The model under review builds one solid part; all positions refer to its coordinate system, in mm. Face numbers are marked on the shaded views. A direction names the side the tool comes from. Round coordinates to 2 decimals unless told otherwise and drop trailing zeros. Write each loop counter-clockwise with the first axis right and the second up, starting at its lowest first coordinate (ties: lowest second). Pieces come first, ordered by that corner, then holes. Notation, with made-up numbers: (71.5, -8) -> (111.5, -8) arc R12 cw to (111.5, 8) -> close; hole circle Ø1 at (73.25, 16). An arc over 180 degrees is marked (long way). Return JSON: item names as keys, results as strings. Group by question number.
1. Mouldability with a two-part tool opening along X and no side actions: class the marked faces 4, 5 and 6 as pulls with the +X half, pulls with the -X half, needs draft (parallel to the pull), parting line crosses it, or undercut.
2. Clearance check with flat-ended pins moving along their axes: P1, Ø8, axis at x = -21.5, y = 5, coming from the -Z side; P2, Ø5.5, axis at x = 24, z = 38, coming from the +Y side; P3, Ø8, axis at x = 21, y = 24.5, coming from the -Z side; P4, Ø0.9, axis at x = -5.5, z = 2, coming from the +Y side. State where each tip first meets the part, or that it passes through.
3. Take a section at D-D, the plane z = 20.5. Write out the cut boundary in (x, y).
4. Take a section at B-B, the plane y = 0. Write out the cut boundary in (x, z).
5. Take a section at A-A, the plane x = 23.25. Write out the cut boundary in (y, z).
6. For line 1 along X through (y, z) = (6.5, 9); line 2 along Y through (x, z) = (23.25, 38.3); line 3 along Y through (x, z) = (-22.25, 36.1), list the stretches that pass through material, from the lowest coordinate up. Write a range as from..to.
7. Tool access review of the marked faces 1, 2 and 3: name each direction out of +Z, -Z, +X, -X, +Y, -Y from which nothing blocks a thin tool from reaching the whole face with its end or side.
8. Take a section at C-C, the plane z = 7.5. Write out the cut boundary in (x, y).
Autodesk Inventor part; units mm, degrees
ref_plane "YZ Plane" through (0, 0, 0) normal (1, 0, 0) x (0, 1, 0)
ref_plane "XZ Plane" through (0, 0, 0) normal (0, 1, 0) x (-1, 0, 0)
ref_plane "XY Plane" through (0, 0, 0) normal (0, 0, 1) x (1, 0, 0)
sketch "Sketch1" plane through (0, 0, 0) normal (0, 0, 1) x (1, 0, 0)
  point P0 (0, 0)
sketch "Sketch2" plane through (0, 0, 0) normal (0, 0, 1) x (1, 0, 0)
  line L0 (-14.25, -53.5) -> (14.25, -53.5)
  line L1 (14.25, -53.5) -> (14.25, 53.5)
  line L2 (14.25, 53.5) -> (-14.25, 53.5)
  line L3 (-14.25, 53.5) -> (-14.25, -53.5)
  line L4 (-14.25, -53.5) -> (14.25, 53.5) construction
  line L5 (14.25, -53.5) -> (-14.25, 53.5) construction
  line L6 (14.25, -53.5) -> (17.25, -53.5)
  line L7 (17.25, -53.5) -> (17.25, 53.5)
  line L8 (17.25, 53.5) -> (14.25, 53.5)
  line L9 (14.25, 53.5) -> (14.25, -53.5)
  line L10 (-14.25, -53.5) -> (-17.25, -53.5)
  line L11 (-17.25, -53.5) -> (-17.25, 53.5)
  line L12 (-17.25, 53.5) -> (-14.25, 53.5)
  line L13 (-14.25, 53.5) -> (-14.25, -53.5)
  line L14 (-17.25, 53.5) -> (17.25, 53.5)
  line L15 (17.25, 53.5) -> (17.25, 56.5)
  line L16 (17.25, 56.5) -> (-17.25, 56.5)
  line L17 (-17.25, 56.5) -> (-17.25, 53.5)
  point P0 (0, 0)
  dimension "d0" = 28.5
  dimension "d1" = 107
  dimension "d2" = 3
  dimension "d3" = 3
  dimension "d4" = 107
  dimension "d5" = 3
extrude "Extrusion1" add sketch "Sketch2" along normal blind 40 contours L10 L11 L12 L3 | L1 L8 L7 L6 | L12 L17 L16 L15 L8 L2
extrude "Extrusion2" add sketch "Sketch2" along normal blind 3 contours L3 L2 L1 L0
ref_plane "Work Plane1" through (-17.25, -53.5, 0) normal (-1, 0, 0) x (0, 0, 1)
sketch "Sketch3" plane through (-17.25, -53.5, 0) normal (-1, 0, 0) x (0, 0, 1)
  line L0 (0, 110) -> (40, 110)
  line L1 (0, 0) -> (40, 0)
  line L2 (40, 110) -> (35, 110)
  line L3 (35, 110) -> (35, 0)
  line L4 (35, 0) -> (40, 0)
  line L5 (40, 0) -> (40, 110)
  point P0 (0, 53.5)
  dimension "d11" = 5
extrude "Extrusion3" add sketch "Sketch3" along normal blind 10
ref_plane "Work Plane2" through (17.25, -53.5, 0) normal (1, 0, 0) x (0, 0, -1)
sketch "Sketch4" plane through (17.25, -53.5, 0) normal (1, 0, 0) x (0, 0, -1)
  line L0 (-40, 0) -> (-40, 110)
  line L1 (-40, 0) -> (-35, 0)
  line L2 (-35, 0) -> (-35, 108.8698)
  line L3 (-35, 108.8698) -> (-40, 108.8698)
  line L4 (-40, 108.8698) -> (-40, 0)
  point P0 (0, 53.5)
  dimension "d15" = 5
extrude "Extrusion4" add sketch "Sketch4" along normal blind 10
ref_plane "Work Plane3" through (-14.25, 53.5, 40) normal (0, -1, 0) x (1, 0, 0)
sketch "Sketch5" plane through (-14.25, 53.5, 40) normal (0, -1, 0) x (1, 0, 0)
  line L0 (0, -37) -> (28.5, -37)
  line L1 (28.5, -37) -> (28.5, 0)
  line L2 (0, -37) -> (28.5, -37)
  line L3 (28.5, -37) -> (28.5, -22)
  line L4 (28.5, -22) -> (0, -22)
  line L5 (0, -22) -> (0, -37)
  line L6 (31.5, 0) -> (-13, 0)
  line L7 (0, 0) -> (28.5, 0)
  line L8 (28.5, 0) -> (28.5, -10)
  line L9 (28.5, -10) -> (0, -10)
  line L10 (0, -10) -> (0, 0)
  point P0 (14.25, -40)
  dimension "d19" = 15
  dimension "d20" = 10
extrude "Extrusion5" cut sketch "Sketch5" against normal blind 10 contours L5 L4 L1 L0
extrude "Extrusion6" cut sketch "Sketch5" against normal blind 10 contours L9 L10 L6 L1
ref_plane "Work Plane4" through (0, 0, 0) normal (0, 0, -1) x (-1, 0, 0)
sketch "Sketch6" plane through (0, 0, 0) normal (0, 0, -1) x (-1, 0, 0)
  line L0 (-14.25, 53.5) -> (-14.25, 56.5)
  line L1 (14.25, -53.5) -> (14.25, 56.5)
  line L2 (-14.25, 56.5) -> (14.25, 56.5)
  line L3 (14.25, 56.5) -> (14.25, 46.5)
  line L4 (14.25, 46.5) -> (-14.25, 46.5)
  line L5 (-14.25, 46.5) -> (-14.25, 56.5)
  point P0 (0, 0)
  point P1 (14.25, 56.5)
  dimension "d26" = 10
extrude "Extrusion7" cut sketch "Sketch6" against normal blind 10
ref_plane "Work Plane5" through (0, 0, 40) normal (0, 0, 1) x (1, 0, 0)
ref_plane "Work Plane6" through (0, 0, 40) normal (0, 0, 1) x (1, 0, 0)
sketch "Sketch7" plane through (0, 0, 40) normal (0, 0, 1) x (1, 0, 0)
  circle A0 centre (23.25, 0) radius 1.75
  point P0 (0, 0)
  dimension "d31" = 3.5
sketch "Sketch8" plane through (0, 0, 40) normal (0, 0, 1) x (1, 0, 0)
  circle A0 centre (-22.25, 0) radius 1.75
  point P0 (0, 0)
  dimension "d32" = 3.5
extrude "Extrusion8" cut sketch "Sketch8" against normal blind 10
extrude "Extrusion9" cut sketch "Sketch7" against normal blind 10
properties part number "suport_batterie_2"
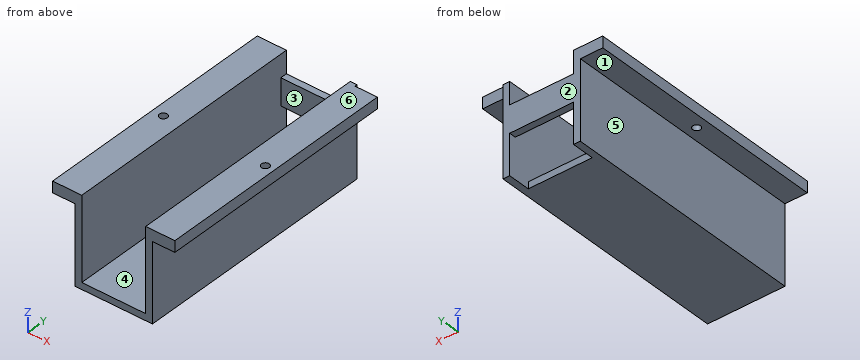
Output:
{
 "1": {"face 4": "undercut", "face 5": "pulls with the -X half", "face 6": "needs draft"},
 "2": {"P1": "stops at z = 35", "P2": "stops at y = 55.37", "P3": "stops at z = 0", "P4": "stops at y = 46.5"},
 "3": {"outline": "(-17.25, -53.5) -> (-14.25, -53.5) -> (-14.25, 53.5) -> (14.25, 53.5) -> (14.25, -53.5) -> (17.25, -53.5) -> (17.25, 56.5) -> (-17.25, 56.5) -> close"},
 "4": {"outline": "(-27.25, 35) -> (-24, 35) -> (-24, 40) -> (-27.25, 40) -> close; (-20.5, 35) -> (-17.25, 35) -> (-17.25, 0) -> (17.25, 0) -> (17.25, 35) -> (21.5, 35) -> (21.5, 40) -> (14.25, 40) -> (14.25, 3) -> (-14.25, 3) -> (-14.25, 40) -> (-20.5, 40) -> close; (25, 35) -> (27.25, 35) -> (27.25, 40) -> (25, 40) -> close"},
 "5": {"outline": "(-53.5, 35) -> (-1.75, 35) -> (-1.75, 40) -> (-53.5, 40) -> close; (1.75, 35) -> (55.37, 35) -> (55.37, 40) -> (1.75, 40) -> close"},
 "6": {"line 1": "x = -17.25..-14.25, 14.25..17.25", "line 2": "y = -53.5..-1.75, 1.75..55.37", "line 3": "y = -53.5..-1.75, 1.75..56.5"},
 "7": {"face 1": "-Z, -X, +Y, -Y", "face 2": "+Z, -Z, +X, -X, +Y", "face 3": "+Z, -Z, -Y"},
 "8": {"outline": "(-17.25, -53.5) -> (-14.25, -53.5) -> (-14.25, 56.5) -> (-17.25, 56.5) -> close; (14.25, -53.5) -> (17.25, -53.5) -> (17.25, 56.5) -> (14.25, 56.5) -> close"}
}
